from build123d import *

# Parameters (mm, degrees)
BOSS_EXTRUDE1_DEPTH = 15
SKETCH2_R           = 2.75
CUT_EXTRUDE1_DEPTH  = 3
SKETCH3_R           = 1.35
CUT_EXTRUDE2_DEPTH  = 9
SKETCH4_R           = 4.05
CUT_EXTRUDE3_DEPTH  = 16


with BuildPart() as part:
    # Sketch1 → Boss-Extrude1 (new body)
    with BuildSketch(Plane.XY):
        with BuildLine():
            Line((0.700840098, 16.455896919), (0.810681557, 6.255896919))
            ThreePointArc((0.810681557, 6.255896919), (5.886159138, 8.587996721), (11.010681557, 6.365738378))
            Line((11.010681557, 6.365738378), (10.900840098, 16.565738378))
            Line((10.900840098, 16.565738378), (0.700840098, 16.455896919))
        make_face()
        with BuildLine():
            ThreePointArc((11.010681557, 6.365738378), (5.886159138, 8.587996721), (0.810681557, 6.255896919))
            Line((0.810681557, 6.255896919), (11.010681557, 6.365738378))
        make_face()
        with BuildLine():
            Line((11.010681557, 6.365738378), (0.810681557, 6.255896919))
            ThreePointArc((0.810681557, 6.255896919), (3.546395485, -4.672331118), (12.809920939, 1.738393871))
            ThreePointArc((12.809920939, 1.738393871), (12.344285051, 4.220811017), (11.010681557, 6.365738378))
        make_face()
    extrude(amount=BOSS_EXTRUDE1_DEPTH)

    # Sketch2 → Cut-Extrude1 (cut)
    with BuildSketch(Plane(origin=(-0.177107964, 16.446442498, 0), x_dir=(0.999942022, 0.010768146, 0), z_dir=(-0.010768146, 0.999942022, 0))):
        with Locations((5.96903182, -7.499323697)):
            Circle(SKETCH2_R)
    extrude(amount=-CUT_EXTRUDE1_DEPTH, mode=Mode.SUBTRACT)

    # Sketch3 → Cut-Extrude2 (cut)
    with BuildSketch(Plane(origin=(-0.144803526, 13.446616432, 0), x_dir=(0.999942022, 0.010768146, 0), z_dir=(-0.010768146, 0.999942022, 0))):
        with Locations((5.96903182, -7.499323697)):
            Circle(SKETCH3_R)
    extrude(amount=-CUT_EXTRUDE2_DEPTH, mode=Mode.SUBTRACT)

    # Sketch4 → Cut-Extrude3 (cut, through all)
    with BuildSketch(Plane(origin=(0, 0, 0), x_dir=(-1, 0, 0), z_dir=(0, 0, -1))):
        with Locations((-5.959920939, 1.738393871)):
            Circle(SKETCH4_R)
    extrude(amount=-CUT_EXTRUDE3_DEPTH, mode=Mode.SUBTRACT)


solid = part.part
Geometry: final body of the model. Coordinates: model frame, mm. A direction names the side the tool comes from. Give positions to 0.01 mm unless a question says otherwise; leave off trailing zeros. Loops run counter-clockwise (first coordinate to the right, second up) from the corner with the lowest first, then second, coordinate; pieces in that order, holes last. Notation, with made-up numbers: M -12,34 L 16,34 A25 cw 16,71 Z; hole C 20,45.5 d8. An arc over 180 degrees is marked long. Put each result on its own line as item: value.
1) Reachability of faces 1 (the cylindrical face through (6.838, -2.215, 7.395)), 2 (the cylindrical face through (6.59, 9.6, 6.36)) from +Z, -Z, +X, -X, +Y, -Y: full face, straight path, thin tool, end or side. Return the list, or none.
Computed values:
face 1: +Z, -Z
face 2: none
2) Material intervals for L1, parallel to X at y = 4, z = 7; L2, parallel to Y at x = 5.75, z = 14; L3, parallel to Y at x = 9.25, z = 13.5, sorted ascending. Write a range as from..to.
Computed values:
L1: x = -0.51..2.6, 9.32..12.43
L2: y = -5.11..-2.31, 5.78..16.51
L3: y = -4.27..-0.62, 4.1..16.55
3) Cut plane C-C, the plane z = 10.5. Return the cut outline in (x, y), plus the area to 3 significant figures.
Computed values:
outline: M 0.7,16.46 L 0.81,6.26 A6.85 ccw long 11.01,6.37 L 10.9,16.57 Z; hole C 5.96,1.74 d8.1
area: 184 mm^2
4) First-contact query: P1, Ø7.5, axis at x = 5.96, y = 1.74, coming from the +Z side; P2, Ø1.5, axis at y = 6, z = 4.5, coming from the -X side; P3, Ø1.5, axis at y = 6.5, z = 13, coming from the +X side; P4, Ø1, axis at y = -1, z = 4.5, coming from the +X side. Flat tips, straight axial feed; report the tip coordinate or a pass-through.
Computed values:
P1: passes through
P2: stops at x = 0.08
P3: stops at x = 11.51
P4: stops at x = 12.43
5) Mould query, pull axis Z, two halves, no side actions, for faces 3 (the cylindrical face through (5.45, 15.028, 4.773)), 4 (the flat face through (6, 6, 15)), 5 (the flat face through (6, 6, 0)). Classes: released by +Z, released by -Z, zero draft, split by the parting line, or undercut.
Computed values:
face 3: undercut
face 4: released by +Z
face 5: released by -Z
6) Cut plane D-D, the plane x = 6.75. Give the number of separate pieces and of enclosed holes in the cut face, plus the area to 3 significant figures.
Computed values:
separate pieces: 3
enclosed holes: 0
area: 173 mm^2
7) Cut plane B-B, the plane x = 2.5. Return the cut outline in (y, z), plus the area to 3 significant figures.
Computed values:
outline: M -4.17,0 L -0.37,0 L -0.37,15 L -4.17,15 Z; M 3.84,0 L 16.48,0 L 16.48,15 L 3.84,15 Z
area: 247 mm^2
8) Cut plane A-A, the plane y = 1.25. Return the cut outline in (x, z).
Computed values:
outline: M -0.87,0 L 1.94,0 L 1.94,15 L -0.87,15 Z; M 9.98,0 L 12.79,0 L 12.79,15 L 9.98,15 Z
